Verification items for the finished model (mm, model axes). A direction names the side the tool comes from. Give positions to 0.01 mm unless a question says otherwise; leave off trailing zeros. Write each loop counter-clockwise with the first axis right and the second up, starting at its lowest first coordinate (ties: lowest second). Pieces come first, ordered by that corner, then holes. Notation, with made-up numbers: (36.5, 75.5) -> (72.5, 75.5) arc R7 cw to (72.5, 82.5) -> close; hole circle Ø11 at (51, 87). An arc over 180 degrees is marked (long way). Answer as CSV lines item,"result". Start each with the question number.
1) Material ranges on L1, parallel to X at y = 8, z = 24.5; L2, parallel to Y at x = -8.25, z = 23; L3, parallel to X at y = 0.75, z = 42.5, recorded low to high.
2) Mould release check, pull along Z, two halves, no side actions. Record for faces 4 (the flat face through (2.732, 0, 26)), 5 (the flat face through (-0.12, 8.08, 44.84)), 6 (the flat face through (0, 0, 0)): released by +Z, released by -Z, zero draft, split by the parting line, or undercut.
3) Tool access check on faces 1 (the flat face through (-2.732, 0, 26)), 2 (the flat face through (-4, 8.724, 24)), 3 (the flat face through (-4, -8.724, 24)). Record the directions out of +Z, -Z, +X, -X, +Y, -Y that give a thin tool (end or side, any length) a straight path to the whole face; none if there is none.
4) Sectioned sample at B-B on z = 22.5. Record the cut outline in (x, y), and give its area (3 significant figures).
5) Gauge pin test, flat ends, axial feed: pin 1 Ø4 at (y, z) = (2.5, 34) entering from -X; pin 2 Ø8.5 at (x, z) = (1.5, 29) entering from -Y; pin 3 Ø8.5 at (x, z) = (-0.5, 25.5) entering from +Y. Record the tip position at first contact, or that the pin passes through.
6) Sectioned sample at C-C on x = 5. Record the cut outline in (y, z).
7) Sectioned sample at D-D on x = 1.5. Record the cut outline in (y, z).
```python
from build123d import *

# Parameters (mm, degrees)
F0_W        = 25.3882817924
F0_H        = 25.3883041441
F1_DEPTH    = 5.08
F2_W        = 17.0946475118
F2_H        = 17.4471139908
F3_DEPTH    = 45.466
F5_DEPTH    = 25.4
F6_DEPTH    = 25.4
F7_SIZE     = 1.27
F8_SIZE     = 1.27
F9_T1_DEPTH = 33.2988026177
F9_T3_DEPTH = 33.2988249694


# Not quite as in the source:
# - a fillet or chamfer that OpenCascade refuses, or shapes differently, is made with other operations: its cross-section is extruded or revolved along the edge and cut away or added


with BuildPart() as f1:
    # F0 (on Top) → F1 (new body)
    with BuildSketch(Plane.XY):
        Rectangle(F0_W, F0_H)
    extrude(amount=F1_DEPTH)

    # F2 (on Top) → F3 (join)
    with BuildSketch(Plane.XY):
        Rectangle(F2_W, F2_H)
    extrude(amount=F3_DEPTH)

    # F4 (on Front) → F5 (cut)
    with BuildSketch(Plane.XZ):
        with BuildLine():
            ThreePointArc((-2.7316187043, 20.3549675643), (-1.8326762864, 18.6002154817), (0.0056849059, 17.8876984864))
            Line((0.0056849059, 17.8876984864), (0.0386628839, 17.8876984864))
            ThreePointArc((0.0386628839, 17.8876984864), (1.7712415134, 18.5095830103), (2.7316187043, 20.0800112066))
            Line((2.7316187043, 20.0800112066), (2.7316187043, 21.236134693))
            Line((2.7316187043, 21.236134693), (2.7316187043, 30.2240438759))
            Line((2.7316187043, 30.2240438759), (2.7316187043, 30.752742663))
            ThreePointArc((2.7316187043, 30.752742663), (2.1863530417, 32.1452825707), (0.9908690064, 33.0437812954))
            Line((0.9908690064, 33.0437812954), (-0.9794991946, 33.0437812954))
            ThreePointArc((-0.9794991946, 33.0437812954), (-2.2272694516, 32.0741140874), (-2.7316187043, 30.5765103549))
            Line((-2.7316187043, 30.5765103549), (-2.7316187043, 30.4002761841))
            Line((-2.7316187043, 30.4002761841), (-2.7316187043, 20.9611783353))
            Line((-2.7316187043, 20.9611783353), (-2.7316187043, 20.3549675643))
        make_face()
        with BuildLine():
            ThreePointArc((-2.7316187043, 20.9611783353), (-2.7482496384, 20.6580729498), (-2.7316187043, 20.3549675643))
            Line((-2.7316187043, 20.3549675643), (-2.7316187043, 20.9611783353))
        make_face()
        with BuildLine():
            Line((2.7316187043, 21.236134693), (2.7316187043, 20.0800112066))
            ThreePointArc((2.7316187043, 20.0800112066), (2.7925974282, 20.6580729498), (2.7316187043, 21.236134693))
        make_face()
        with BuildLine():
            ThreePointArc((-2.7316187043, 30.5765103549), (-2.7330366343, 30.4883932695), (-2.7316187043, 30.4002761841))
            Line((-2.7316187043, 30.4002761841), (-2.7316187043, 30.5765103549))
        make_face()
        with BuildLine():
            Line((2.7316187043, 30.752742663), (2.7316187043, 30.2240438759))
            ThreePointArc((2.7316187043, 30.2240438759), (2.7444064461, 30.4883932695), (2.7316187043, 30.752742663))
        make_face()
        with BuildLine():
            ThreePointArc((0.9908690064, 33.0437812954), (0.0056849059, 33.2271148097), (-0.9794991946, 33.0437812954))
            Line((-0.9794991946, 33.0437812954), (0.9908690064, 33.0437812954))
        make_face()
    extrude(amount=-F5_DEPTH, mode=Mode.SUBTRACT)

    # F6 (cut): a face of the model
    f6_faces = [f1.faces().sort_by_distance(p)[0] for p in [
        (0.0051043388, 0, 25.5481593175),
    ]]
    extrude(f6_faces, amount=-F6_DEPTH, mode=Mode.SUBTRACT)

    # F7
    f7_edges = [f1.edges().sort_by_distance(p)[0] for p in [
        (0, -12.694152, 0),
        (12.694141, 0, 0),
        (-12.694141, 0, 0),
        (0, 12.694152, 0),
    ]]
    chamfer(f7_edges, length=F7_SIZE)

    # F8
    f8_edges = [f1.edges().sort_by_distance(p)[0] for p in [
        (0, 8.723557, 45.466),
        (-8.547324, 0, 45.466),
        (0, -8.723557, 45.466),
        (8.547324, 0, 45.466),
    ]]
    chamfer(f8_edges, length=F8_SIZE)

    # F9: fillet of radius 5.08 on 4 edges, made by hand

    # F9_s2 → F9_t1 (cut)
    with BuildSketch(Plane.YZ.offset(-16.6494013088)):
        with BuildLine():
            ThreePointArc((-12.6941520721, 1.27), (-11.1300991312, 0.3280951188), (-9.334047907, 0))
            Line((-9.334047907, 0), (-11.4241520721, 0))
            Line((-11.4241520721, 0), (-12.6941520721, 1.27))
        make_face()
        with BuildLine():
            ThreePointArc((12.6941520721, 1.27), (11.1300991312, 0.3280951188), (9.334047907, 0))
            Line((9.334047907, 0), (11.4241520721, 0))
            Line((11.4241520721, 0), (12.6941520721, 1.27))
        make_face()
    extrude(amount=F9_T1_DEPTH, mode=Mode.SUBTRACT)

    # F9_s4 → F9_t3 (cut)
    with BuildSketch(Plane.XZ.offset(-16.6494124847)):
        with BuildLine():
            ThreePointArc((12.6941408962, 1.27), (11.1300879554, 0.3280951188), (9.3340367311, 0))
            Line((9.3340367311, 0), (11.4241408962, 0))
            Line((11.4241408962, 0), (12.6941408962, 1.27))
        make_face()
        with BuildLine():
            ThreePointArc((-12.6941408962, 1.27), (-11.1300879554, 0.3280951188), (-9.3340367311, 0))
            Line((-9.3340367311, 0), (-11.4241408962, 0))
            Line((-11.4241408962, 0), (-12.6941408962, 1.27))
        make_face()
    extrude(amount=F9_T3_DEPTH, mode=Mode.SUBTRACT)


solid = f1.part
```
Ans:
1,L1,"x = -8.55 to -2.73, 2.73 to 8.55"
1,L2,"y = -8.72 to 8.72"
1,L3,"x = -8.55 to 8.55"
2,face 4,"undercut"
2,face 5,"released by +Z"
2,face 6,"released by -Z"
3,face 1,"+Y, -Y"
3,face 2,"+Z, +X, -X, +Y"
3,face 3,"+Z, +X, -X, -Y"
4,outline,"(-8.55, -8.72) -> (-2.73, -8.72) -> (-2.73, 8.72) -> (-8.55, 8.72) -> close; (2.73, -8.72) -> (8.55, -8.72) -> (8.55, 8.72) -> (2.73, 8.72) -> close"
4,area,"203 mm²"
5,pin 1,"stops at x = -8.55"
5,pin 2,"stops at y = -8.72"
5,pin 3,"stops at y = 8.72"
6,outline,"(-12.69, 1.27) arc R5.08 ccw to (-9.33, 0) -> (9.33, 0) arc R5.08 ccw to (12.69, 1.27) -> (12.69, 5.08) -> (8.72, 5.08) -> (8.72, 44.2) -> (7.45, 45.47) -> (-7.45, 45.47) -> (-8.72, 44.2) -> (-8.72, 5.08) -> (-12.69, 5.08) -> close"
7,outline,"(-12.69, 1.27) arc R5.08 ccw to (-9.33, 0) -> (9.33, 0) arc R5.08 ccw to (12.69, 1.27) -> (12.69, 5.08) -> (8.72, 5.08) -> (8.72, 18.31) -> (-8.72, 18.31) -> (-8.72, 5.08) -> (-12.69, 5.08) -> close; (-8.72, 32.78) -> (8.72, 32.78) -> (8.72, 44.2) -> (7.45, 45.47) -> (-7.45, 45.47) -> (-8.72, 44.2) -> close"
